Part print with two shaded views. Sizes in mm from the minimum x, y, z corner. Round coordinates to 2 decimals unless told otherwise and drop trailing zeros. Loops run counter-clockwise (first coordinate to the right, second up) from the corner with the lowest first, then second, coordinate; pieces in that order, holes last. Notation, with made-up numbers: (29, 87.25) - (79, 87.25) arc R28 ccw to (79, 106.25) - close; hole circle Ø5 at (70, 78). An arc over 180 degrees is marked (long way). One line per question, with ' | ' between items.
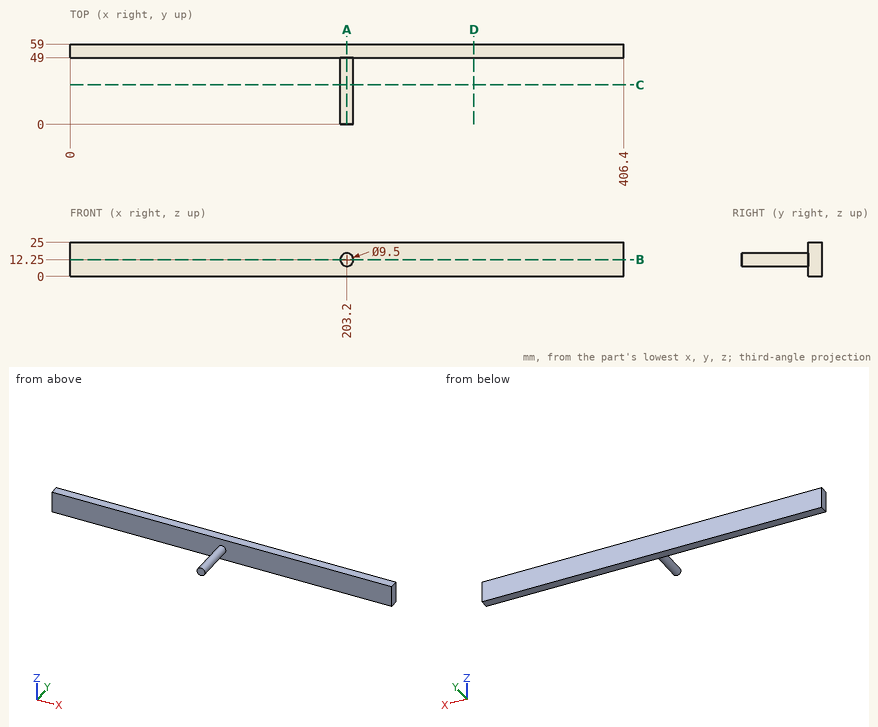
(1) Cut at D-D, the plane x = 296.5. Write the cut outline in (y, z).
Results found:
outline: (49, 0) - (59, 0) - (59, 25) - (49, 25) - close
(2) Drop flat-ended pins along their axis: P1, Ø3, axis at x = 148.5, z = 8, coming from the -Y side; P2, Ø6, axis at y = 14.5, z = 18, coming from the -X side; P3, Ø4, axis at y = 27.5, z = 12, coming from the +X side. Give the stop position or say it passes through.
Results found:
P1: stops at y = 49 | P2: stops at x = 199.33 | P3: stops at x = 207.95
(3) Cut at B-B, the plane z = 12.25. Write the cut outline in (x, y).
Results found:
outline: (0, 49) - (198.45, 49) - (198.45, 0) - (207.95, 0) - (207.95, 49) - (406.4, 49) - (406.4, 59) - (0, 59) - close
(4) Probe L1, parallel to Y at x = 107, z = 16; L2, parallel to X at y = 23.5, z = 12; L3, parallel to X at y = 44, z = 14.5. List the from-to ranges inside material, lowest first.
Results found:
L1: y = 49 to 59 | L2: x = 198.46 to 207.94 | L3: x = 199.02 to 207.38
(5) Cut at C-C, the plane y = 29. Write the cut outline in (x, z).
Results found:
outline: circle Ø9.5 at (203.2, 12.25)
(6) Cut at A-A, the plane x = 203.2. Write the cut outline in (y, z).
Results found:
outline: (0, 7.5) - (49, 7.5) - (49, 0) - (59, 0) - (59, 25) - (49, 25) - (49, 17) - (0, 17) - close
